Read the model definition and answer for the solid it produces. Units are mm, in the model's axes. Face numbers are marked on the shaded views. A direction names the side the tool comes from. Coordinates: 2 decimals unless noted, no trailing zeros. Write each loop counter-clockwise with the first axis right and the second up, starting at its lowest first coordinate (ties: lowest second). Pieces come first, ordered by that corner, then holes. Notation, with made-up numbers: (57.25, 61) - (102.25, 61) arc R18 cw to (102.25, 89) - close; hole circle Ø8 at (37.5, 73.25). An arc over 180 degrees is marked (long way). Return JSON: item names as keys, results as strings.
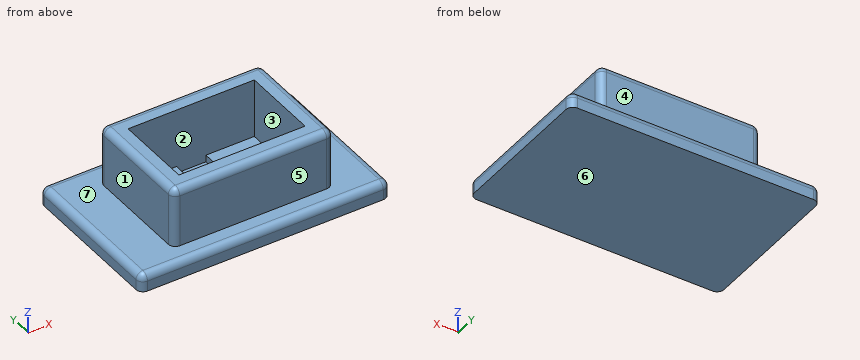
```python
from build123d import *

# Parameters (mm, degrees)
F0_W     = 36.5
F0_H     = 22.5
F1_DEPTH = 17
F2_T     = 5
F3_W     = 8.5
F3_H     = 22.5
F4_DEPTH = 2
F0_W_2   = 72.2177475691
F0_H_2   = 44.6370989084
F5_DEPTH = 5
F6_R     = 2


# Not quite as in the source:
# - two fillets or chamfers of one size are made in one step


with BuildPart() as f1:
    # F0 (on Top) → F1 (new body)
    with BuildSketch(Plane.XY):
        with Locations((0.1048383191, -0.5443561636)):
            Rectangle(F0_W, F0_H)
    extrude(amount=F1_DEPTH)

    # F2
    f2_openings = [f1.faces().sort_by_distance(p)[0] for p in [
        (0.104838, -0.544356, 17),
    ]]
    offset(amount=F2_T, openings=f2_openings, kind=Kind.INTERSECTION)

    # F3 (on face) → F4 (cut)
    with BuildSketch(Plane.XY):
        with Locations((0.1048383191, -0.5443561636)):
            Rectangle(F3_W, F3_H)
    extrude(amount=-F4_DEPTH, mode=Mode.SUBTRACT)

    # F0 (on Top) → F5 (join)
    with BuildSketch(Plane.XY):
        Rectangle(F0_W_2, F0_H_2)
        with Locations((0.1048383191, -0.5443561636)):
            Rectangle(F0_W, F0_H, mode=Mode.SUBTRACT)
    extrude(amount=-F5_DEPTH)

    # F6
    f6_edges = [f1.edges().sort_by_distance(p)[0] for p in [
        (36.108874, -22.318549, -2.5),
        (36.108874, 22.318549, -2.5),
        (-36.108874, -22.318549, -2.5),
        (-36.108874, 22.318549, -2.5),
        (-23.145162, -0.544356, 17),
        (0.104838, -16.794356, 17),
        (23.354838, -0.544356, 17),
        (0.104838, 15.705644, 17),
        (-23.145162, -16.794356, 8.5),
        (-23.145162, 15.705644, 8.5),
        (23.354838, -16.794356, 8.5),
        (23.354838, 15.705644, 8.5),
        (0, 22.318549, 0),
        (36.108874, 0, 0),
        (-36.108874, 0, 0),
        (0, -22.318549, 0),
    ]]
    fillet(f6_edges, radius=F6_R)


solid = f1.part
```
(1) A cutting plane is placed at B-B (y = 2). Determine the outline of the cut face in (x, z).
Answer:
{"outline": "(-36.11, -5) - (36.11, -5) - (36.11, -2) arc R2 ccw to (34.11, 0) - (23.35, 0) - (23.35, 15) arc R2 ccw to (21.35, 17) - (18.35, 17) - (18.35, 0) - (4.35, 0) - (4.35, -2) - (-4.15, -2) - (-4.15, 0) - (-18.15, 0) - (-18.15, 17) - (-21.15, 17) arc R2 ccw to (-23.15, 15) - (-23.15, 0) - (-34.11, 0) arc R2 ccw to (-36.11, -2) - close"}
(2) Determine the mould class of the marked faces 1, 2, 3 and 4 for opening direction X: +X half, -X half, draft (parallel to the pull), parting line (faces both ways), or undercut.
Answer:
{"face 1": "-X half", "face 2": "undercut", "face 3": "undercut", "face 4": "draft"}
(3) Straight lines are drawn through the part: line 1 (X direction, y = -3.5, z = 12.75); line 2 (Y direction, x = -2.5, z = 10.75); line 3 (X direction, y = -6.5, z = 15.25). For each, find the intervals that lie inside material, in ascending order. Write a range as from..to.
Answer:
{"line 1": "-23.15..-18.15, 18.35..23.35", "line 2": "-16.79..-11.79, 10.71..15.71", "line 3": "-23.13..-18.15, 18.35..23.34"}
(4) Which of the six approach directions +Z, -Z, +X, -X, +Y, -Y give full straight-line access (tool end or side, diameter ignored) to the marked faces 5, 6 and 7?
Answer:
{"face 5": "+Z, +X, -X, -Y", "face 6": "-Z, +X, -X, +Y, -Y", "face 7": "+Z"}
(5) A cutting plane is placed at D-D (x = -24.5). Determine the outline of the cut face in (y, z).
Answer:
{"outline": "(-22.32, -5) - (22.32, -5) - (22.32, -2) arc R2 ccw to (20.32, 0) - (-20.32, 0) arc R2 ccw to (-22.32, -2) - close"}
(6) Flat-ended cylindrical pins translate along their axes: P1, Ø1.5, axis at y = 9, z = 11.5, coming from the +X side; P2, Ø4.5, axis at x = 7, z = 10.5, coming from the +Y side; P3, Ø2, axis at x = 7.5, z = 9.5, coming from the -Y side. Find the tip coordinate at first contact, or state that the pin passes through.
Answer:
{"P1": "x = 23.35", "P2": "y = 15.71", "P3": "y = -16.79"}
(7) A cutting plane is placed at C-C (z = 3.5). Determine the outline of the cut face in (x, y), and give its area (3 significant figures).
Answer:
{"outline": "(-23.15, -14.79) arc R2 ccw to (-21.15, -16.79) - (21.35, -16.79) arc R2 ccw to (23.35, -14.79) - (23.35, 13.71) arc R2 ccw to (21.35, 15.71) - (-21.15, 15.71) arc R2 ccw to (-23.15, 13.71) - close; hole (-18.15, -11.79) - (18.35, -11.79) - (18.35, 10.71) - (-18.15, 10.71) - close", "area": "687 mm²"}
(8) A cutting plane is placed at A-A (x = -13). Determine the outline of the cut face in (y, z).
Answer:
{"outline": "(-22.32, -5) - (22.32, -5) - (22.32, -2) arc R2 ccw to (20.32, 0) - (15.71, 0) - (15.71, 15) arc R2 ccw to (13.71, 17) - (10.71, 17) - (10.71, 0) - (-11.79, 0) - (-11.79, 17) - (-14.79, 17) arc R2 ccw to (-16.79, 15) - (-16.79, 0) - (-20.32, 0) arc R2 ccw to (-22.32, -2) - close"}
